```python
from build123d import *

# Parameters (mm, degrees)
F0_W            = 12.7
F0_H            = 50.8
F2_W            = 5.08
F2_H            = 50.5912028922
F3_DEPTH        = 6.35
F3_DEPTH_BACK   = 6.35
F3_COPIES_COUNT = 6
F4_R            = 6.6777820133
F5_DEPTH        = 25.4
F5_COPIES_COUNT = 6
F7_W            = 6.35
F7_H            = 101.6


# Not quite as in the source:
# - a pattern or mirror of a feature is missing from the dataset's text; its kind, count and spacing are read off the source's solid


with BuildPart() as f1:
    # F0 (on Front) → F1 (revolve)
    with BuildSketch(Plane.XZ):
        with Locations((-34.29, 25.4)):
            Rectangle(F0_W, F0_H)
    revolve(axis=Axis((0, 0, 19.3039998412), (0, 0, 1)))

    # F2 (on Front) → F3 (join, two sides)
    with BuildSketch(Plane.XZ) as f3_sk:
        with BuildLine():
            Line((-40.64, 0), (-40.64, 50.5912028922))
            ThreePointArc((-40.64, 50.5912028922), (-63.7394462668, 25.2956014461), (-40.64, 0))
        make_face()
        with Locations((-38.1, 25.2956014461)):
            Rectangle(F2_W, F2_H)
    f3 = extrude(amount=F3_DEPTH) + extrude(f3_sk.sketch, amount=-F3_DEPTH_BACK)

    # F3_copies: F3 ×6 about axis
    f3_copies_axis = Axis((0, 0, 0), (0, 0, 1))
    for i in range(1, F3_COPIES_COUNT):
        add(f3.rotate(f3_copies_axis, i * 360 / F3_COPIES_COUNT))

    # F4 (on face) → F5 (cut)
    with BuildSketch(Plane.XZ.offset(6.35)):
        with Locations((-52.8408407984, 25.4)):
            Circle(F4_R)
    f5 = extrude(amount=-F5_DEPTH, mode=Mode.SUBTRACT)

    # F5_copies: F5 ×6 about axis
    f5_copies_axis = Axis((0, 0, 0), (0, 0, 1))
    for i in range(1, F5_COPIES_COUNT):
        add(f5.rotate(f5_copies_axis, i * 360 / F5_COPIES_COUNT), mode=Mode.SUBTRACT)

    # F7 (on Front) → F8 (revolve)
    with BuildSketch(Plane.XZ):
        with Locations((-31.115, 25.4)):
            Rectangle(F7_W, F7_H)
    revolve(axis=Axis((0, 0, 73.8201290369), (0, 0, 1)))


solid = f1.part
```
Check sheet for the modelled part. Datum: model origin and axes. Units: mm. A direction names the side the tool comes from. Round coordinates to 2 decimals unless told otherwise and drop trailing zeros. Loops run counter-clockwise (first coordinate to the right, second up) from the corner with the lowest first, then second, coordinate; pieces in that order, holes last. Notation, with made-up numbers: (-16.75, -22) - (-2.75, -22) arc R22 ccw to (-2.75, -5) - close; hole circle Ø1 at (26.25, 23). An arc over 180 degrees is marked (long way). Answer as a JSON object with one key per item and string values. Group by question number.
Q1. Sectioned sample at C-C, the plane z = 25.4. Count the separate pieces of the cut face and the enclosed holes in it, plus the area to 3 significant figures.
Q2. Sectioned sample at B-B, the plane z = 45.5. Enter the section's corners in (x, y).
Q3. Scan lines: line 1 along Y through (x, z) = (0, 4); line 2 along X through (y, z) = (0, 25); line 3 along X through (y, z) = (3, 25). Record each from-to range of solid material in increasing order. Write a range as [from, to].
Q4. Set-up check for faces 1 (the face through (16.62, -41.49, 25.65)), 2 (the face through (-44, -6.35, 26)), 3 (the face through (-27.62, -35.14, 25.65)), 4 (the face through (-44, 6.35, 26)), 5 (the face through (24.7, -42.61, 31.03)): record each of +Z, -Z, +X, -X, +Y, -Y from which the full face is reachable in a straight line by a thin tool's end or side.
Q5. Sectioned sample at A-A, the plane x = 0. Enter the section's corners in (y, z).
Q6. Mould release check, pull along Y, two halves, no side actions. Record for faces 6 (the face through (24, 25, 0)), 7 (the face through (-24.7, 42.61, 31.03)), 8 (the face through (31.79, -55.24, 25.82)): released by +Y, released by -Y, zero draft, split by the parting line, or undercut.
Q7. Gauge pin test, flat ends, axial feed: P1, Ø3.5, axis at x = -17.5, y = 37, coming from the +Z side; P2, Ø6, axis at x = 27, y = -37, coming from the +Z side; P3, Ø10, axis at x = -39.5, z = 64.5, coming from the -Y side; P4, Ø6, axis at x = 18.5, z = 42.5, coming from the -Y side. Record the tip position at first contact, or that the pin passes through.
Q8. Sectioned sample at D-D, the plane z = 66. Enter the section's corners in (x, y), plus the area to 3 significant figures.
Solution:
{
 "1": {"separate pieces": "7", "enclosed holes": "1", "area": "3,490 mm²"},
 "2": {"outline": "(-53.73, -6.35) - (-40.14, -6.35) arc R40.64 ccw to (-25.57, -31.59) - (-32.37, -43.36) - (-21.37, -49.71) - (-14.57, -37.94) arc R40.64 ccw to (14.57, -37.94) - (21.37, -49.71) - (32.37, -43.36) - (25.57, -31.59) arc R40.64 ccw to (40.14, -6.35) - (53.73, -6.35) - (53.73, 6.35) - (40.14, 6.35) arc R40.64 ccw to (25.57, 31.59) - (32.37, 43.36) - (21.37, 49.71) - (14.57, 37.94) arc R40.64 ccw to (-14.57, 37.94) - (-21.37, 49.71) - (-32.37, 43.36) - (-25.57, 31.59) arc R40.64 ccw to (-40.14, 6.35) - (-53.73, 6.35) - close; hole circle Ø55.88 at (0, 0)"},
 "3": {"line 1": "y = [-40.64, -27.94], [27.94, 40.64]", "line 2": "x = [-63.74, -59.51], [-46.18, -27.94], [27.94, 46.18], [59.51, 63.74]", "line 3": "x = [-63.74, -59.51], [-46.18, -27.78], [27.78, 46.18], [59.51, 63.74]"},
 "4": {"face 1": "+Z, -Z, -Y", "face 2": "+Z, -Z, -X, -Y", "face 3": "+Z, -Z, -X", "face 4": "+Z, -Z, -X, +Y", "face 5": "none"},
 "5": {"outline": "(-40.64, 0) - (-34.29, 0) - (-34.29, -25.4) - (-27.94, -25.4) - (-27.94, 76.2) - (-34.29, 76.2) - (-34.29, 50.8) - (-40.64, 50.8) - close; (27.94, -25.4) - (34.29, -25.4) - (34.29, 0) - (40.64, 0) - (40.64, 50.8) - (34.29, 50.8) - (34.29, 76.2) - (27.94, 76.2) - close"},
 "6": {"face 6": "zero draft", "face 7": "undercut", "face 8": "released by -Y"},
 "7": {"P1": "stops at z = 50.8", "P2": "stops at z = 50.35", "P3": "passes through", "P4": "stops at y = -49.94"},
 "8": {"outline": "circle Ø68.58 at (0, 0); hole circle Ø55.88 at (0, 0)", "area": "1,240 mm²"}
}
